from build123d import *

# Parameters (mm, degrees)
BOSS_EXTRUDE1_DEPTH = 28
SKETCH2_R           = 1
CUT_EXTRUDE1_DEPTH  = 8


with BuildPart() as part:
    # Sketch1 → Boss-Extrude1 (new body)
    with BuildSketch(Plane.XY):
        with BuildLine():
            Line((2.091427576, 20.661862086), (19.061990324, 3.691299338))
            add(Edge.make_bspline(
                [(19.061990324, 3.691299338), (12.022648732, 1.181374363), (3.606718166, -4.502881384), (-8.768521596, -14.578433411), (-15.710250584, -19.650895957), (-19.63487909, -24.098483284)],
                knots=[0, 0, 0, 0, 0.463104191, 0.631300778, 1, 1, 1, 1], degree=3))
            add(Edge.make_bspline(
                [(-19.63487909, -24.098483284), (-25.969562098, -30.737294566), (-30.045502317, -42.502143037)],
                knots=[0, 0, 0, 1, 1, 1], degree=2))
            Line((-30.045502317, -42.502143037), (-32.987873718, -42.502143037))
            add(Edge.make_bspline(
                [(2.091427576, 20.661862086), (-6.153665282, 13.902778077), (-14.884492863, 1.613682443), (-29.203935151, -18.642558282), (-31.728248971, -33.20873178), (-32.987873718, -42.502143037)],
                knots=[0, 0, 0, 0, 0.426775149, 0.611805153, 1, 1, 1, 1], degree=3))
        make_face()
    extrude(amount=BOSS_EXTRUDE1_DEPTH)

    # Sketch2 → Cut-Extrude1 (cut)
    with BuildSketch(Plane(origin=(11.376644831, 11.376644831, 0), x_dir=(0, 0, -1), z_dir=(0.7071067811865388, 0.7071067811865562, 0))):
        with Locations(Location((-7, 1.131280172, 0), (0, 0, 90))):
            Circle(SKETCH2_R)
        with Locations(Location((-14, 8.131280172, 0), (0, 0, 270))):
            Circle(SKETCH2_R)
        with Locations(Location((-14, -5.868719828, 0), (0, 0, 90))):
            Circle(SKETCH2_R)
        with Locations(Location((-21, 1.131280172, 0), (0, 0, 270))):
            Circle(SKETCH2_R)
    extrude(amount=-CUT_EXTRUDE1_DEPTH, mode=Mode.SUBTRACT)


solid = part.part
Source: CAD feature listing. Evaluate the final solid. Frame: model axes, mm. A direction names the side the tool comes from. Round coordinates to 2 decimals unless told otherwise and drop trailing zeros. Return JSON: item names as keys, results as strings. Group by question number.
1. Mould query, pull axis Z, two halves, no side actions, for faces 3 (the face through (-31, -42.502, 14)), 4 (the face through (-9, -4, 0)), 5 (the face through (7.88, 9.3, 7.99)), 6 (the face through (4.91, 6.53, 20.99)). Classes: released by +Z, released by -Z, zero draft, split by the parting line, or undercut.
2. Pin query (flat end, axial travel): pin 1 (12 mm diameter, centred on x = -18.5, z = 8.5, fed in from -Y); pin 2 (3 mm diameter, centred on x = 5, z = 22.5, fed in from -Y); pin 3 (5 mm diameter, centred on x = -19.5, z = 3, fed in from +Y). Return the tip coordinate at first contact, or that it passes through.
3. Reachability of faces 1 (the face through (-0.04, 11.48, 13.99)), 2 (the face through (-9, -4, 28)) from +Z, -Z, +X, -X, +Y, -Y: full face, straight path, thin tool, end or side. Return the list, or none.
4. Material intervals for line 1 along Y through (x, z) = (12, 14.25); line 2 along X through (y, z) = (12.5, 11.5); line 3 along X through (y, z) = (-26.5, 3.25), sorted ascending. Write a range as from..to.
Checks:
{
 "1": {"face 3": "zero draft", "face 4": "released by -Z", "face 5": "undercut", "face 6": "undercut"},
 "2": {"pin 1": "stops at y = -30.49", "pin 2": "stops at y = -4.89", "pin 3": "stops at y = -1.39"},
 "3": {"face 1": "none", "face 2": "+Z, +X, -X, +Y, -Y"},
 "4": {"line 1": "y = 0.52..2.33, 5.07..10.75", "line 2": "x = -6.29..10.25", "line 3": "x = -30.02..-21.72"}
}
